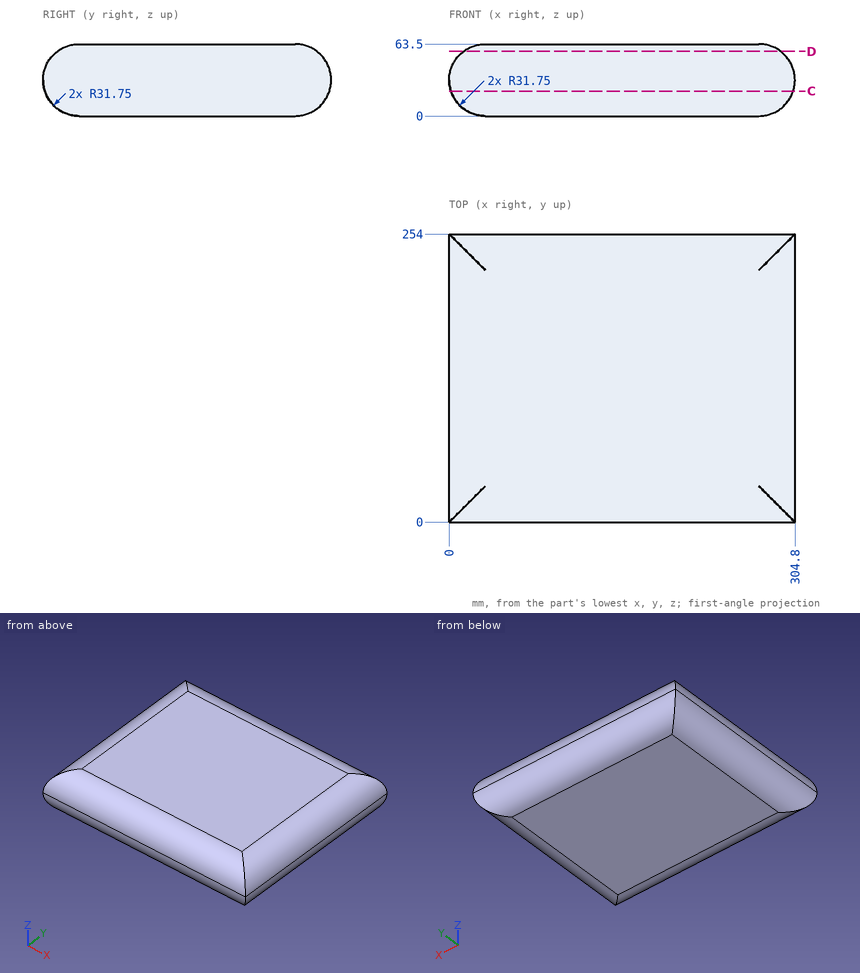
Check sheet for the drawn part. Datum: minimum x, y, z corner. Units: mm. Coordinates: 2 decimals unless noted, no trailing zeros. Loops run counter-clockwise (first coordinate to the right, second up) from the corner with the lowest first, then second, coordinate; pieces in that order, holes last. Notation, with made-up numbers: (-14, -38) -> (-9, -38) arc R15 ccw to (-9, -24) -> close; hole circle Ø4 at (-33.75, -15). An arc over 180 degrees is marked (long way). Answer in a Markdown table with one row per item.
1) Section check C-C (z = 22). Record the cut outline in (x, y), and give its area (3 significant figures).
The answers:
| item | result |
|---|---|
| outline | (1.53, 1.53) -> (303.27, 1.53) -> (303.27, 252.47) -> (1.53, 252.47) -> close |
| area | 75,700 mm2 |
2) Depth check by flat-ended pin: P1, Ø8, axis at y = 142, z = 7, coming from the +X side; P2, Ø1.5, axis at y = 155, z = 33, coming from the -X side; P3, Ø8, axis at x = 176.5, z = 9, coming from the +Y side. Enter the tip coordinate at first touch or a pass-through.
The answers:
| item | result |
|---|---|
| P1 | stops at x = 297.08 |
| P2 | stops at x = 0 |
| P3 | stops at y = 247.87 |
3) Scan lines: line 1 along Z through (x, y) = (275, 140); line 2 along Y through (x, z) = (236, 38.5); line 3 along X through (y, z) = (150, 11). Record each from-to range of solid material in increasing order. Write a range as from..to.
The answers:
| item | result |
|---|---|
| line 1 | z = 0.06..63.44 |
| line 2 | y = 0.73..253.27 |
| line 3 | x = 7.72..297.08 |
4) Section check D-D (z = 57). Record the cut outline in (x, y), and give its area (3 significant figures).
The answers:
| item | result |
|---|---|
| outline | (12.5, 12.5) -> (292.3, 12.5) -> (292.3, 241.5) -> (12.5, 241.5) -> close |
| area | 64,100 mm2 |
